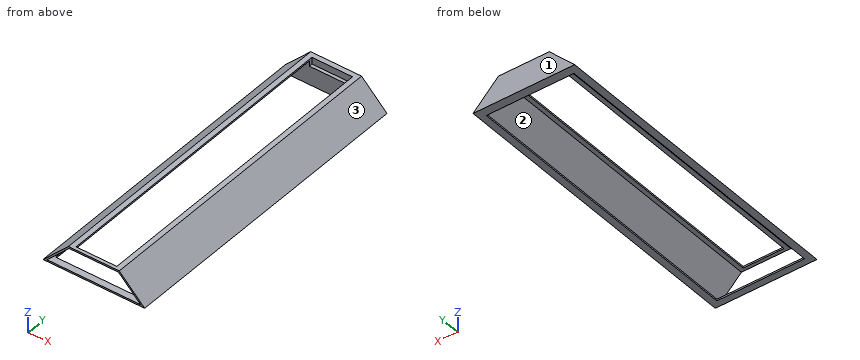
Autodesk Fusion 360 part; units mm, degrees
sketch "top hopper side" plane through (0, 0, 0) normal (0, 1, 0) x (1, 0, 0)
  line L0 (-76.2, 0) -> (0, 0)
  line L1 (0, 0) -> (-19.05, -19.05)
  line L2 (-19.05, -19.05) -> (-57.15, -19.05)
  line L3 (-57.15, -19.05) -> (-76.2, 0)
  dimension "d12" = 76.2
  dimension "d13" = 38.1
  dimension "d14" = 45
extrude "Extrude3" add sketch "top hopper side" along normal blind 234.95
sketch "side cutout" plane through (0, 0, 0) normal (0, -1, 0) x (1, 0, 0)
  line L0 (-19.05, 19.05) -> (-57.15, 19.05)
  line L1 (-57.15, 19.05) -> (-76.2, 0)
  line L2 (-76.2, 0) -> (0, 0)
  line L3 (0, 0) -> (-19.05, 19.05)
  line L4 (-76.2, 0) -> (-57.15, 19.05)
  line L5 (-19.05, 19.05) -> (0, 0)
  line L6 (-76.2, 0) -> (0, 0)
  line L7 (-57.15, 19.05) -> (-19.05, 19.05)
  line L8 (-73.1339, 1.27) -> (-3.0661, 1.27)
  line L9 (-19.5761, 17.78) -> (-3.0661, 1.27)
  line L10 (-56.6239, 17.78) -> (-19.5761, 17.78)
  line L11 (-73.1339, 1.27) -> (-56.6239, 17.78)
  dimension "d17" = 1.27
extrude "Extrude4" cut sketch "side cutout" against normal blind 228.6 contours L8 L9 L10 L11
sketch "bottom cutout" plane through (0, 0, 0) normal (0, 0, -1) x (1, 0, 0)
  line L0 (0, 0) -> (-76.2, 0)
  line L1 (-76.2, 0) -> (-76.2, -234.95)
  line L2 (-76.2, -234.95) -> (0, -234.95)
  line L3 (0, -234.95) -> (0, 0)
  line L4 (-5.08, -5.08) -> (-70.7474, -5.08)
  line L5 (-70.7474, -5.08) -> (-70.7474, -228.6)
  line L6 (-5.08, -228.6) -> (-5.08, -5.08)
  line L7 (-5.08, -228.6) -> (-70.7474, -228.6)
  dimension "d20" = 223.52
  dimension "d21" = 65.6674
  dimension "d22" = 5.08
  dimension "d23" = 5.08
extrude "Extrude5" cut sketch "bottom cutout" against normal blind 2.54 contours L4 L5 L6 L7
sketch "top cutout" plane through (0, 0, 19.05) normal (0, 0, 1) x (-1, 0, 0)
  line L0 (57.15, 0) -> (19.05, 0)
  line L1 (19.05, 0) -> (19.05, -234.95)
  line L2 (19.05, -234.95) -> (57.15, -234.95)
  line L3 (57.15, -234.95) -> (57.15, 0)
  line L4 (53.34, -2.54) -> (22.86, -2.54)
  line L5 (22.86, -2.54) -> (22.86, -231.14)
  line L6 (22.86, -231.14) -> (53.34, -231.14)
  line L7 (53.34, -231.14) -> (53.34, -2.54)
  dimension "d26" = 228.6
  dimension "d27" = 30.48
  dimension "d28" = 3.81
  dimension "d29" = 2.54
extrude "Extrude6" cut sketch "top cutout" against normal blind 5.08 contours L4 L5 L6 L7
Here's how the part is built. I have some questions about the finished solid (model axes, mm). Face numbers are marked on the shaded views. Coordinates: 2 decimals unless noted, no trailing zeros. Order: outer loops, then holes, each group sorted by start corner. A loop starts at its lowest first (then second) coordinate and runs counter-clockwise, first axis right, second up. Notation, with made-up numbers: M -3,32.25 L 17,32.25 A22 cw 17,68.25 Z; hole C 48.25,12.25 d4. An arc over 180 degrees is marked long. Answer as a JSON object with one key per item and string values. Group by question number.
(1) Suppose I cut it at C-C, the plane z = 5.25. Please give me the cut outline in (x, y), then the cut area to 3 significant figures.
(2) Suppose I cut it at B-B, the plane x = -36. Please give me the cut outline in (y, z).
(3) Suppose I cut it at A-A, the plane y = 182.5. Please give me the cut outline in (x, z), then the cut area to 3 significant figures.
(4) If we mould it in two halves opening along X, with no side actions, what happens to the marked faces 1, 2 and 3? For each: released by +X, released by -X, zero draft, split by the parting line, or undercut.
(5) For pin 1 (2 mm diameter, centred on x = -52, y = 112.5, fed in from +Z); pin 2 (3 mm diameter, centred on y = 139.5, z = 15.5, fed in from +X); pin 3 (2 mm diameter, centred on x = -14.5, z = 9.5, fed in from -Y); pin 4 (5.5 mm diameter, centred on y = 106.5, z = 17, fed in from -X), each with a flat end and sliding along its axis, tell me the tip position at first contact or that it passes through.
(6) I need wall thicknesses on probe 1 along Y at (x, z) = (-70, 2.75); probe 2 along X at (y, z) = (71, 4); probe 3 along X at (y, z) = (145.5, 2.5). Which ranges of each line are inside material? Lowest first, please.
Values found:
{
 "1": {"outline": "M -70.95,0 L -69.15,0 L -69.15,228.6 L -7.05,228.6 L -7.05,0 L -5.25,0 L -5.25,234.95 L -70.95,234.95 Z", "area": "1,240 mm^2"},
 "2": {"outline": "M 0,0 L 5.08,0 L 5.08,1.27 L 0,1.27 Z; M 0,17.78 L 2.54,17.78 L 2.54,19.05 L 0,19.05 Z; M 228.6,0 L 234.95,0 L 234.95,19.05 L 231.14,19.05 L 231.14,13.97 L 228.6,13.97 Z"},
 "3": {"outline": "M -76.2,0 L -70.75,0 L -70.75,1.27 L -73.13,1.27 L -56.62,17.78 L -53.34,17.78 L -53.34,19.05 L -57.15,19.05 Z; M -22.86,17.78 L -19.58,17.78 L -3.07,1.27 L -5.08,1.27 L -5.08,0 L 0,0 L -19.05,19.05 L -22.86,19.05 Z", "area": "82.4 mm^2"},
 "4": {"face 1": "zero draft", "face 2": "undercut", "face 3": "released by +X"},
 "5": {"pin 1": "passes through", "pin 2": "stops at x = -14", "pin 3": "stops at y = 228.6", "pin 4": "stops at x = -61.95"},
 "6": {"probe 1": "y = 228.6 to 234.95", "probe 2": "x = -72.2 to -70.4, -5.8 to -4", "probe 3": "x = -73.7 to -71.9, -4.3 to -2.5"}
}
